Part model, mm, in its own coordinate system. Face numbers are marked on the shaded views. A direction names the side the tool comes from. Round coordinates to 2 decimals unless told otherwise and drop trailing zeros. Loops run counter-clockwise (first coordinate to the right, second up) from the corner with the lowest first, then second, coordinate; pieces in that order, holes last.
1) Band-saw the part on A-A, the plane x = 4.25. Write the cut outline in (y, z).
2) Drop flat-ended pins along their axis: P1, Ø1, axis at x = 3, z = 0.5, coming from the +Y side; P2, Ø1, axis at y = 1.5, z = 6, coming from the +X side; P3, Ø1, axis at x = 0, y = -2, coming from the +Z side. Give the stop position or say it passes through.
3) Band-saw the part on C-C, the plane y = -2.5. Write the cut outline in (x, z), then the cut area to 3 significant figures.
4) 3-axis set-ups, long thin cutter, end or side, ignore diameter. For the marked faces 4, 5 and 6: which of +Z, -Z, +X, -X, +Y, -Y reach the whole face in a straight line?
5) Mould opens along Z. For the marked faces 1, 2 and 3 say: +Z half, -Z half, draft (parallel to the pull), parting line (faces both ways), or undercut.
6) Probe line 1 (Z direction, x = -2, y = 1); line 2 (X direction, y = -0.5, z = 3.75); line 3 (Y direction, x = 0, z = 3.5) (3 decimals). List the from-to ranges inside material, lowest first.
7) Band-saw the part on B-B, the plane z = 4. Write the cut outline in (x, y) (3 decimals), then the cut area to 3 significant figures.
8) Band-saw the part on D-D, the plane x = 0. Write the cut outline in (y, z) (3 decimals).
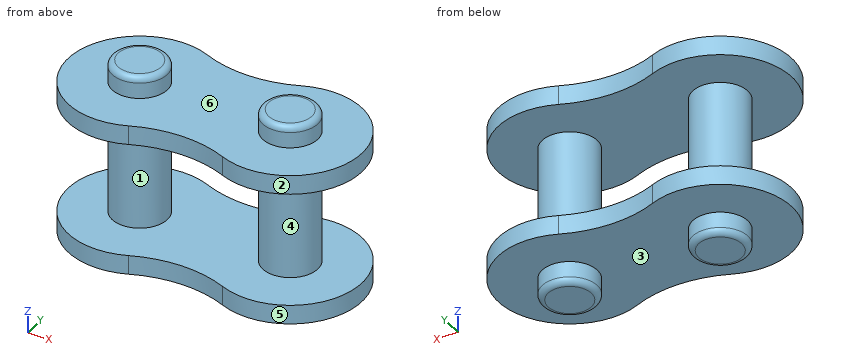
from build123d import *

# Parameters (mm, degrees)
EXTRUDE_1_DEPTH = 0.8
SKETCH_2_R      = 1.155
EXTRUDE_2_DEPTH = 4.78
EXTRUDE_3_DEPTH = 0.8
SKETCH_4_R      = 1.155
EXTRUDE_4_DEPTH = 0.91
EXTRUDE_START   = 0.91
SKETCH_5_R      = 1.155
EXTRUDE_5_DEPTH = 0.91
FILLET_1_R      = 0.25


with BuildPart() as part:
    # 草图1 → 凸台-拉伸1 (new body)
    with BuildSketch(Plane.XY):
        with BuildLine():
            ThreePointArc((1.190625, 2.753618004), (-3, 0), (1.190625, -2.753618004))
            ThreePointArc((1.190625, -2.753618004), (3.175, -2.342981343), (5.159375, -2.753618004))
            ThreePointArc((5.159375, -2.753618004), (9.35, 0), (5.159375, 2.753618004))
            ThreePointArc((5.159375, 2.753618004), (3.175, 2.342981343), (1.190625, 2.753618004))
        make_face()
    extrude(amount=EXTRUDE_1_DEPTH)

    # 草图2 → 凸台-拉伸2 (add)
    with BuildSketch(Plane.XY.offset(0.8)):
        Circle(SKETCH_2_R)
        with Locations((6.35, 0)):
            Circle(SKETCH_2_R)
    extrude(amount=EXTRUDE_2_DEPTH)

    # 草图3 → 凸台-拉伸3 (add)
    with BuildSketch(Plane.XY.offset(5.58)):
        with BuildLine():
            ThreePointArc((5.159375, -2.753618004), (3.175, -2.342981343), (1.190625, -2.753618004))
            ThreePointArc((1.190625, -2.753618004), (-3, 0), (1.190625, 2.753618004))
            ThreePointArc((1.190625, 2.753618004), (3.175, 2.342981343), (5.159375, 2.753618004))
            ThreePointArc((5.159375, 2.753618004), (9.35, 0), (5.159375, -2.753618004))
        make_face()
    extrude(amount=EXTRUDE_3_DEPTH)

    # 草图4 → 凸台-拉伸4 (add)
    with BuildSketch(Plane.XY.offset(6.38)):
        Circle(SKETCH_4_R)
        with Locations((6.35, 0)):
            Circle(SKETCH_4_R)
    extrude(amount=EXTRUDE_4_DEPTH)

    # 草图5 → 凸台-拉伸5 (add)
    with BuildSketch(Plane(origin=(0, 0, 0), x_dir=(-1, 0, 0), z_dir=(0, 0, -1)).offset(EXTRUDE_START)):
        with Locations(Location((0, 0, 0), (0, 0, 180))):
            Circle(SKETCH_5_R)
        with Locations(Location((-6.35, 0, 0), (0, 0, 180))):
            Circle(SKETCH_5_R)
    extrude(amount=-EXTRUDE_5_DEPTH)

    # 圆角1
    fillet_1_edges = [part.edges().sort_by_distance(p)[0] for p in [
        (-1.155, 0, 7.29),
        (5.195, 0, 7.29),
        (-1.155, 0, -0.91),
        (5.195, 0, -0.91),
    ]]
    fillet(fillet_1_edges, radius=FILLET_1_R)


solid = part.part
Reported:
1. outline: (-2.46, 0) - (2.46, 0) - (2.46, 0.8) - (-2.46, 0.8) - close; (-2.46, 5.58) - (2.46, 5.58) - (2.46, 6.38) - (-2.46, 6.38) - close
2. P1: stops at y = 2.39
2. P2: stops at x = 9.18
2. P3: stops at z = 6.38
3. outline: (-1.66, 0) - (1.93, 0) - (1.93, 0.8) - (-1.66, 0.8) - close; (-1.66, 5.58) - (1.93, 5.58) - (1.93, 6.38) - (-1.66, 6.38) - close; (4.42, 0) - (8.01, 0) - (8.01, 0.8) - (4.42, 0.8) - close; (4.42, 5.58) - (8.01, 5.58) - (8.01, 6.38) - (4.42, 6.38) - close
3. area: 11.5 mm2
4. face 4: none
4. face 5: +Z, -Z
4. face 6: +Z
5. face 1: undercut
5. face 2: draft
5. face 3: -Z half
6. line 1: z = 0 to 0.8, 5.58 to 6.38
6. line 2: x = -1.04 to 1.04, 5.31 to 7.39
6. line 3: y = -1.155 to 1.155
7. outline: circle Ø2.31 at (0, 0); circle Ø2.31 at (6.35, 0)
7. area: 8.38 mm2
8. outline: (-3, 0) - (-1.155, 0) - (-1.155, -0.66) arc R0.25 ccw to (-0.905, -0.91) - (0.905, -0.91) arc R0.25 ccw to (1.155, -0.66) - (1.155, 0) - (3, 0) - (3, 0.8) - (1.155, 0.8) - (1.155, 5.58) - (3, 5.58) - (3, 6.38) - (1.155, 6.38) - (1.155, 7.04) arc R0.25 ccw to (0.905, 7.29) - (-0.905, 7.29) arc R0.25 ccw to (-1.155, 7.04) - (-1.155, 6.38) - (-3, 6.38) - (-3, 5.58) - (-1.155, 5.58) - (-1.155, 0.8) - (-3, 0.8) - close
